The figure shows three views and two pictorial views of one solid part (mm, origin at its lowest corner). Answer the questions. Coordinates: 2 decimals unless noted, no trailing zeros. Write each loop counter-clockwise with the first axis right and the second up, starting at its lowest first coordinate (ties: lowest second). Pieces come first, ordered by that corner, then holes. Notation, with made-up numbers: (53.5, 77) - (66.5, 77) arc R31 ccw to (66.5, 114) - close; hole circle Ø7 at (-9.75, 69). An arc over 180 degrees is marked (long way). Use a Markdown table: item, result. Add a question column.
(1) Given pin 1 Ø3 at (x, z) = (160, 12) entering from -Y; pin 2 Ø15 at (x, y) = (97.5, 180) entering from -Z, each flat-ended and moving along its own axis, determine where each tip first touches the part or whether it passes through.
(2) The part is cut by section A-A, the plane x = 97.5. Give the vertices of the cut face in (y, z).
(3) Find the intervals of material crossed by line 1 (Y direction, x = 97.5, z = 12); line 2 (Y direction, x = 100, z = 31); line 3 (X direction, y = 170.5, z = 20), in increasing order. Write a range as from..to.
(4) The part is cut by section B-B, the plane y = 180. Give the vertices of the cut face in (x, z).
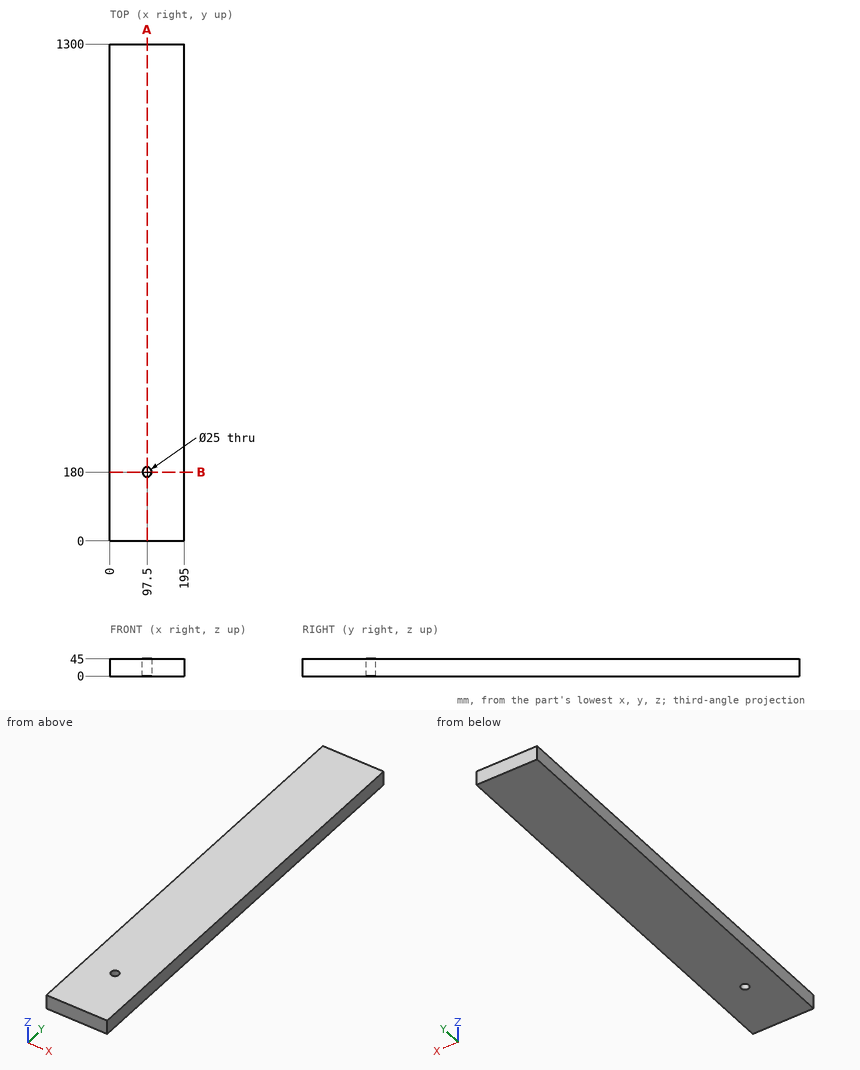
Model answer:
| question | item | result |
|---|---|---|
| 1 | pin 1 | y = 0 |
| 1 | pin 2 | through |
| 2 | outline | (0, 0) - (167.5, 0) - (167.5, 45) - (0, 45) - close; (192.5, 0) - (1300, 0) - (1300, 45) - (192.5, 45) - close |
| 3 | line 1 | 0..167.5, 192.5..1300 |
| 3 | line 2 | 0..167.75, 192.25..1300 |
| 3 | line 3 | 0..89.38, 105.62..195 |
| 4 | outline | (0, 0) - (85, 0) - (85, 45) - (0, 45) - close; (110, 0) - (195, 0) - (195, 45) - (110, 45) - close |
